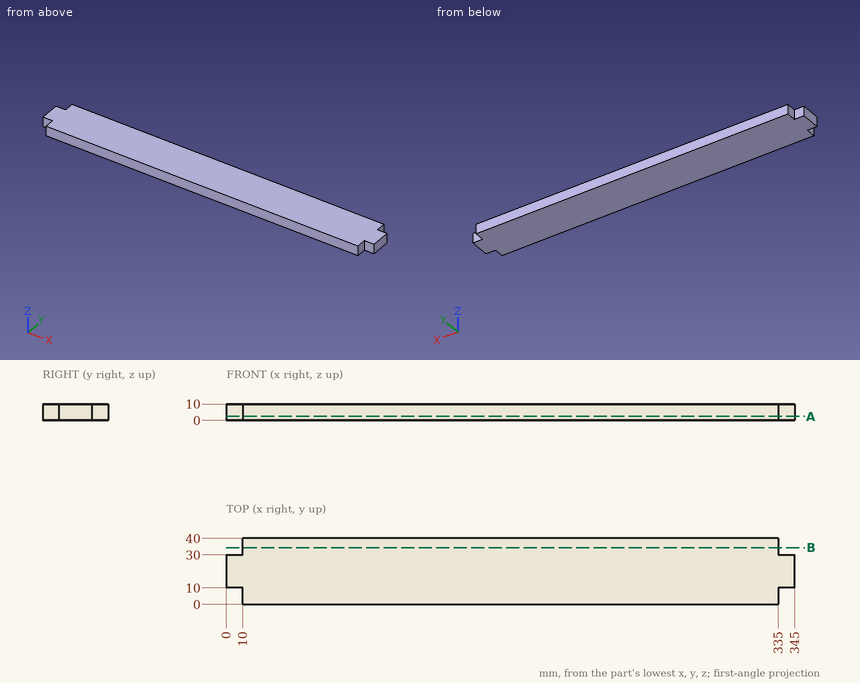
Geometry check sheet. Reference: drawing and pictorial views, mm from the part's lowest x, y, z. Give positions to 0.01 mm unless a question says otherwise; leave off trailing zeros. Loops run counter-clockwise (first coordinate to the right, second up) from the corner with the lowest first, then second, coordinate; pieces in that order, holes last. Notation, with made-up numbers: (86.25, 28.25) - (111.25, 28.25) arc R26 cw to (111.25, 61.25) - close; hole circle Ø7 at (11, 84.25). An arc over 180 degrees is marked (long way). One line per question, with ' | ' between items. Start each with the question number.
1. Gauge pin test, flat ends, axial feed: pin 1 Ø3 at (y, z) = (3, 4) entering from +X; pin 2 Ø3 at (x, z) = (340, 6.5) entering from -Y; pin 3 Ø1 at (y, z) = (31.5, 8) entering from -X. Record the tip position at first contact, or that the pin passes through.
2. Cross-section at B-B, the plane y = 34.5. Enter the section's corners in (x, z), plus the area to 3 significant figures.
3. Material ranges on line 1 along X through (y, z) = (35.5, 7.25), recorded low to high. Write a range as [from, to].
4. Cross-section at A-A, the plane z = 2.5. Enter the section's corners in (x, y), plus the area to 3 significant figures.
Check result:
1) pin 1: stops at x = 335 | pin 2: stops at y = 10 | pin 3: stops at x = 10
2) outline: (10, 0) - (335, 0) - (335, 10) - (10, 10) - close | area: 3,250 mm2
3) line 1: x = [10, 335]
4) outline: (0, 10) - (10, 10) - (10, 0) - (335, 0) - (335, 10) - (345, 10) - (345, 30) - (335, 30) - (335, 40) - (10, 40) - (10, 30) - (0, 30) - close | area: 13,400 mm2
